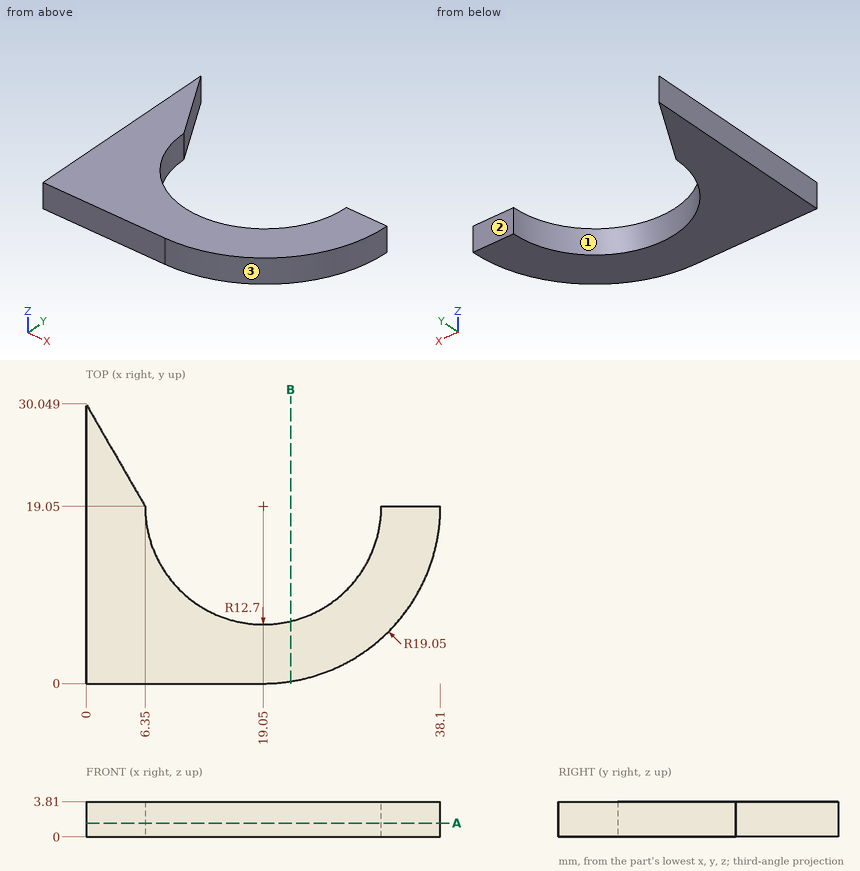
Can you work these out from the drawing? Everything is in mm from the part's minimum corner. Coordinates: 2 decimals unless noted, no trailing zeros. Order: outer loops, then holes, each group sorted by start corner. A loop starts at its lowest first (then second) coordinate and runs counter-clockwise, first axis right, second up. Notation, with made-up numbers: (25, 76) -> (60, 76) arc R15 cw to (60, 105) -> close; hole circle Ø7 at (55, 43). An arc over 180 degrees is marked (long way). Return JSON: item names as keys, results as strings.
1) If I drill on probe 1 along Y at (x, z) = (19.5, 2.7) (1 decimal); probe 2 along X at (y, z) = (15.5, 2.5) (1 decimal); probe 3 along X at (y, z) = (10.5, 0.5) (1 decimal), over which ranges is the centre line in solid material (lowest first)?
Conclusion:
{"probe 1": "y = 0 to 6.4", "probe 2": "x = 0 to 6.9, 31.2 to 37.8", "probe 3": "x = 0 to 9.7, 28.4 to 36.1"}
2) If we section it at B-B on x = 22: List the corners of the cut face in (y, z) for me.
Conclusion:
{"outline": "(0.23, 0) -> (6.7, 0) -> (6.7, 3.81) -> (0.23, 3.81) -> close"}
3) I'm going to push flat-ended pins straight in: P1, Ø12, axis at x = 12, y = 17.5, coming from the -Z side; P2, Ø1.9, axis at x = 34.5, z = 2.5, coming from the +Y side. Where does each tip first touch, or does it pass through?
Conclusion:
{"P1": "stops at z = 0", "P2": "stops at y = 19.05"}
4) Thinking about a two-plate mould opening in X: for the marked faces 1, 2 and 3, which applies, +X half, -X half, draft (parallel to the pull), parting line (faces both ways), or undercut?
Conclusion:
{"face 1": "undercut", "face 2": "draft", "face 3": "+X half"}
5) If we section it at A-A on z = 1.5: List the corners of the cut face in (x, y) for me.
Conclusion:
{"outline": "(0, 0) -> (19.05, 0) arc R19.05 ccw to (38.1, 19.05) -> (31.75, 19.05) arc R12.7 cw to (6.35, 19.05) -> (0, 30.05) -> close"}
